from build123d import *

# Parameters (mm, degrees)
SKETCH2_W                = 500
SKETCH2_H                = 450
BOSS_EXTRUDE1_DEPTH      = 800
BOSS_EXTRUDE1_DEPTH_BACK = 200
CHAMFER1_SIZE            = 20
CHAMFER1_SIZE2           = 200
CHAMFER2_SIZE            = 20
CHAMFER2_SIZE2           = 120
SKETCH9_W                = 317.816050667
SKETCH9_H                = 80.00001522
BOSS_EXTRUDE2_DEPTH      = 300
SKETCH10_W               = 283.451852853
SKETCH10_H               = 161.628693338
CUT_EXTRUDE1_DEPTH       = 10
SKETCH11_R               = 20
CUT_EXTRUDE2_DEPTH       = 10
SKETCH12_W               = 152.997678588
SKETCH12_H               = 274.954886326
CUT_EXTRUDE3_DEPTH       = 10
SKETCH13_W               = 152.997678588
SKETCH13_H               = 17.889097052
BOSS_EXTRUDE3_DEPTH      = 175
SKETCH15_W               = 402.299842062
SKETCH15_H               = 272.648708127
CUT_EXTRUDE4_DEPTH       = 70


with BuildPart() as part:
    # Sketch2 → Boss-Extrude1 (new body, two sides)
    with BuildSketch(Plane(origin=(0, 0, 0), x_dir=(1, 0, 0), z_dir=(0, 1, 0))) as boss_extrude1_sk:
        Rectangle(SKETCH2_W, SKETCH2_H)
    extrude(amount=BOSS_EXTRUDE1_DEPTH)
    extrude(boss_extrude1_sk.sketch, amount=-BOSS_EXTRUDE1_DEPTH_BACK)

    # Chamfer1
    chamfer1_edges = [part.edges().sort_by_distance(p)[0] for p in [
        (0, 800, 225),
    ]]
    chamfer1_side = [part.faces().sort_by_distance(p)[0] for p in [
        (0, 300, 225),
    ]]
    chamfer(chamfer1_edges, length=CHAMFER1_SIZE, length2=CHAMFER1_SIZE2, reference=chamfer1_side[0])

    # Chamfer2
    chamfer2_edges = [part.edges().sort_by_distance(p)[0] for p in [
        (0, 800, -225),
    ]]
    chamfer2_side = [part.faces().sort_by_distance(p)[0] for p in [
        (0, 300, -225),
    ]]
    chamfer(chamfer2_edges, length=CHAMFER2_SIZE, length2=CHAMFER2_SIZE2, reference=chamfer2_side[0])

    # Sketch9 → Boss-Extrude2 (add)
    with BuildSketch(Plane(origin=(0, 800, 0), x_dir=(1, 0, 0), z_dir=(0, 1, 0))):
        with Locations((-91.091974667, 64.99999239)):
            Rectangle(SKETCH9_W, SKETCH9_H)
        Polygon((250, 105), (67.816050667, 105), (67.816050667, 24.99998478), (67.816050667, 8.908040554), (250, 8.908040554), align=None)
    extrude(amount=BOSS_EXTRUDE2_DEPTH)

    # Sketch10 → Cut-Extrude1 (cut)
    with BuildSketch(Plane.XY.offset(-24.99998478)):
        with Locations((-91.091974667, 900)):
            Rectangle(SKETCH10_W, SKETCH10_H)
    extrude(amount=-CUT_EXTRUDE1_DEPTH, mode=Mode.SUBTRACT)

    # Sketch11 → Cut-Extrude2 (cut)
    with BuildSketch(Plane.XY.offset(225)):
        with Locations((110.472474251, 164.751161956)):
            Circle(SKETCH11_R)
        with Locations((174.967964998, 164.751161956)):
            Circle(SKETCH11_R)
        with Locations((110.472474251, 97.062825132)):
            Circle(SKETCH11_R)
        with Locations((174.967964998, 97.062825132)):
            Circle(SKETCH11_R)
    extrude(amount=-CUT_EXTRUDE2_DEPTH, mode=Mode.SUBTRACT)

    # Sketch12 → Cut-Extrude3 (cut)
    with BuildSketch(Plane.XY.offset(-8.908040554)):
        with Locations((158.466067066, 962.522556837)):
            Rectangle(SKETCH12_W, SKETCH12_H)
    extrude(amount=-CUT_EXTRUDE3_DEPTH, mode=Mode.SUBTRACT)

    # Sketch13 → Boss-Extrude3 (add)
    with BuildSketch(Plane(origin=(0, 825.045113674, 0), x_dir=(1, 0, 0), z_dir=(0, 1, 0))):
        with Locations((158.466067066, 96.055451474)):
            Rectangle(SKETCH13_W, SKETCH13_H)
    extrude(amount=BOSS_EXTRUDE3_DEPTH)

    # Sketch15 → Cut-Extrude4 (cut)
    with BuildSketch(Plane(origin=(0, 0, -225), x_dir=(-1, 0, 0), z_dir=(0, 0, -1))):
        with Locations((0.051547356, -27.71868848)):
            Rectangle(SKETCH15_W, SKETCH15_H)
    extrude(amount=-CUT_EXTRUDE4_DEPTH, mode=Mode.SUBTRACT)


solid = part.part
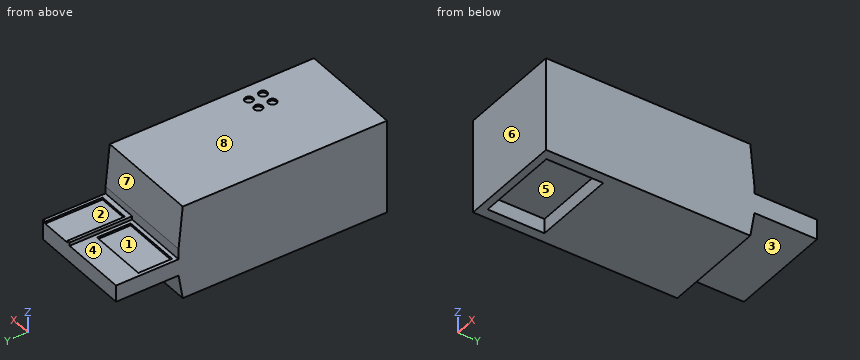
Geometry check sheet. Reference: the model listing, model coordinates, mm. Face numbers are marked on the shaded views. A direction names the side the tool comes from. Round coordinates to 2 decimals unless told otherwise and drop trailing zeros. Write each loop counter-clockwise with the first axis right and the second up, starting at its lowest first coordinate (ties: lowest second). Pieces come first, ordered by that corner, then holes. Notation, with made-up numbers: (-36.75, 59.5) -> (-28.75, 59.5) arc R14 ccw to (-28.75, 76.5) -> close; hole circle Ø3 at (7.25, 29). An arc over 180 degrees is marked (long way). One line per item, written item: value. Start each with the question number.
(1) Cross-section at D-D, the plane y = 958.5. Record the cut outline in (x, z), and give its area (3 significant figures).
(2) Go/stop test with flat-tipped pins: pin 1 Ø8 at (x, z) = (-82, 149.5) entering from +Y; pin 2 Ø12 at (x, z) = (179, 10.5) entering from +Y; pin 3 Ø5 at (y, z) = (942, -19) entering from -X. Record where each tip stops, or that it passes through.
(3) Cross-section at A-A, the plane y = -79. Record the cut outline in (x, z).
(4) Cross-section at C-C, the plane z = -170. Record the cut outline in (x, y), and give its area (3 significant figures).
(5) Access from +Z, -Z, +X, -X, +Y, -Y to the whole of each face (thin tool, end or side, straight path). Record for the marked faces 1, 2, 3 and 4.
(6) Draft check along Y on the marked faces 5, 6, 7 and 8. Enter one of: +Y half, -Y half, draft (parallel to the pull), parting line (faces both ways), or undercut.
(7) Cross-section at B-B, the plane x = -150.5. Record the cut outline in (y, z), and give its area (3 significant figures).
(8) Scan lines: line 1 (Z direction, x = 52, y = -104); line 2 (Y direction, x = 172, z = -189); line 3 (Y direction, x = -119.5, z = -13.5). Record each from-to range of solid material in increasing order. Write a range as [from, to].
Answer:
1. outline: (-250, -105) -> (250, -105) -> (250, -8.91) -> (234.96, -8.91) -> (234.96, -18.91) -> (81.97, -18.91) -> (81.97, -8.91) -> (67.82, -8.91) -> (67.82, -25) -> (50.63, -25) -> (50.63, -35) -> (-232.82, -35) -> (-232.82, -25) -> (-250, -25) -> close
1. area: 38,600 mm²
2. pin 1: y = 787.95
2. pin 2: y = 800
2. pin 3: x = 67.82
3. outline: (-250, -225) -> (-201.2, -225) -> (-201.2, -155) -> (201.1, -155) -> (201.1, -225) -> (250, -225) -> (250, 225) -> (-250, 225) -> close
4. outline: (-250, -200) -> (250, -200) -> (250, 789.17) -> (-250, 789.17) -> close; hole (-201.2, -164.04) -> (201.1, -164.04) -> (201.1, 108.61) -> (-201.2, 108.61) -> close
4. area: 385,000 mm²
5. face 1: +Z
5. face 2: +Z, +Y
5. face 3: -Z, +X, -X, +Y
5. face 4: +Z, -X, +Y
6. face 5: undercut
6. face 6: -Y half
6. face 7: +Y half
6. face 8: draft
7. outline: (-200, -225) -> (-164.04, -225) -> (-164.04, -155) -> (108.61, -155) -> (108.61, -225) -> (780, -225) -> (800, -105) -> (1100, -105) -> (1100, -25) -> (980.81, -25) -> (980.81, -35) -> (819.19, -35) -> (819.19, -25) -> (800, -25) -> (800, 25) -> (780, 225) -> (-200, 225) -> close
7. area: 450,000 mm²
8. line 1: [-155, 225]
8. line 2: [-200, -164.04], [108.61, 786]
8. line 3: [-200, 800]
